```python
from build123d import *

# Parameters (mm, degrees)
EXTRUDE_1_DEPTH     = 45
SKETCH_2_R          = 2
CUT_EXTRUDE_1_DEPTH = 10.8
CUT_EXTRUDE_2_DEPTH = 7.8


with BuildPart() as part:
    # Эскиз1 → Бобышка-Вытянуть1 (new body)
    with BuildSketch(Plane(origin=(0, 0, 0), x_dir=(0, 0, -1), z_dir=(1, 0, 0))):
        Polygon((0, 5), (0, 6), (3, 6), (3, 7.8), (0, 7.8), (0, 9.8), (7, 9.8), (7, 0), (0, 0), (-2.25, 0), (-2.25, 5), align=None)
    extrude(amount=EXTRUDE_1_DEPTH)

    # Эскиз2 → Вырез-Вытянуть1 (cut, through all)
    with BuildSketch(Plane(origin=(0, 9.8, 0), x_dir=(1, 0, 0), z_dir=(0, 1, 0))):
        with Locations((5.5, 0.75)):
            Circle(SKETCH_2_R)
        with Locations((39.5, 0.75)):
            Circle(SKETCH_2_R)
    extrude(amount=-CUT_EXTRUDE_1_DEPTH, mode=Mode.SUBTRACT)

    # Эскиз3 → Вырез-Вытянуть2 (cut)
    with BuildSketch(Plane(origin=(0, 9.8, 0), x_dir=(1, 0, 0), z_dir=(0, 1, 0))):
        with BuildLine():
            Line((2.5, 0.75), (2.5, -2.25))
            Line((2.5, -2.25), (8.5, -2.25))
            Line((8.5, -2.25), (8.5, 0.75))
            ThreePointArc((8.5, 0.75), (5.5, 3.75), (2.5, 0.75))
        make_face()
        with BuildLine():
            Line((36.5, 0.75), (36.5, -2.25))
            Line((36.5, -2.25), (42.5, -2.25))
            Line((42.5, -2.25), (42.5, 0.75))
            ThreePointArc((42.5, 0.75), (39.5, 3.75), (36.5, 0.75))
        make_face()
    extrude(amount=-CUT_EXTRUDE_2_DEPTH, mode=Mode.SUBTRACT)


solid = part.part
```
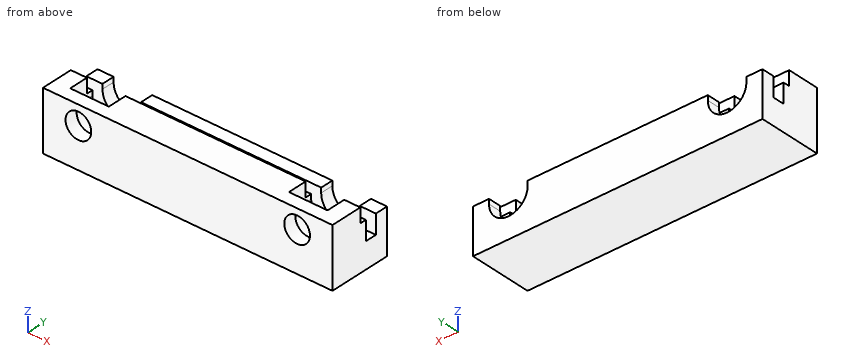
Check sheet for the modelled part. Datum: model origin and axes. Units: mm. Coordinates: 2 decimals unless noted, no trailing zeros. Loops run counter-clockwise (first coordinate to the right, second up) from the corner with the lowest first, then second, coordinate; pieces in that order, holes last.
1) Sectioned sample at B-B (y = 2.5). Record the boundary of the cut face in (x, z), and give its area (3 significant figures).
2) Sectioned sample at D-D (x = 32). Record the boundary of the cut face in (y, z).
3) Sectioned sample at C-C (z = 1.75). Record the boundary of the cut face in (x, y).
4) Sectioned sample at A-A (x = 5.5). Record the boundary of the cut face in (y, z), and give its area (4 significant figures).
5) Material ranges on probe 1 along X at (y, z) = (3.25, 0.5); probe 2 along X at (y, z) = (0.85, -0.75); probe 3 along Y at (x, z) = (15, -2.75), recorded low to high.
6) Gauge pin test, flat ends, axial feed: pin 1 (0.9 mm diameter, centred on x = 22, y = 7, fed in from +Z); pin 2 (0.7 mm diameter, centred on x = 1, z = 1.5, fed in from +Y); pin 3 (2 mm diameter, centred on x = 43.5, y = 8.5, fed in from +Z). Record the tip position at first contact, or that the pin passes through.
Check sheet entries:
1. outline: (0, -7) - (45, -7) - (45, 2.25) - (42.5, 2.25) - (42.5, -0.75) arc R3 cw to (36.5, -0.75) - (36.5, 2.25) - (8.5, 2.25) - (8.5, -0.75) arc R3 cw to (2.5, -0.75) - (2.5, 2.25) - (0, 2.25) - close
1. area: 352 mm2
2. outline: (0, -7) - (9.8, -7) - (9.8, 0) - (7.8, 0) - (7.8, -3) - (6, -3) - (6, 0) - (5, 0) - (5, 2.25) - (0, 2.25) - close
3. outline: (0, 0) - (45, 0) - (45, 5) - (42.5, 5) - (42.5, 2) - (36.5, 2) - (36.5, 5) - (8.5, 5) - (8.5, 2) - (2.5, 2) - (2.5, 5) - (0, 5) - close
4. outline: (0, -7) - (9.8, -7) - (9.8, -3.75) - (2, -3.75) - (2, -2.75) - (0, -2.75) - close; (0, 1.25) - (2, 1.25) - (2, 2.25) - (0, 2.25) - close
4. area: 35.85 mm2
5. probe 1: x = 0 to 2.5, 8.5 to 36.5, 42.5 to 45
5. probe 2: x = 0 to 3.5, 7.5 to 37.5, 41.5 to 45
5. probe 3: y = 0 to 6, 7.8 to 9.8
6. pin 1: stops at z = -3
6. pin 2: stops at y = 5
6. pin 3: stops at z = 0
